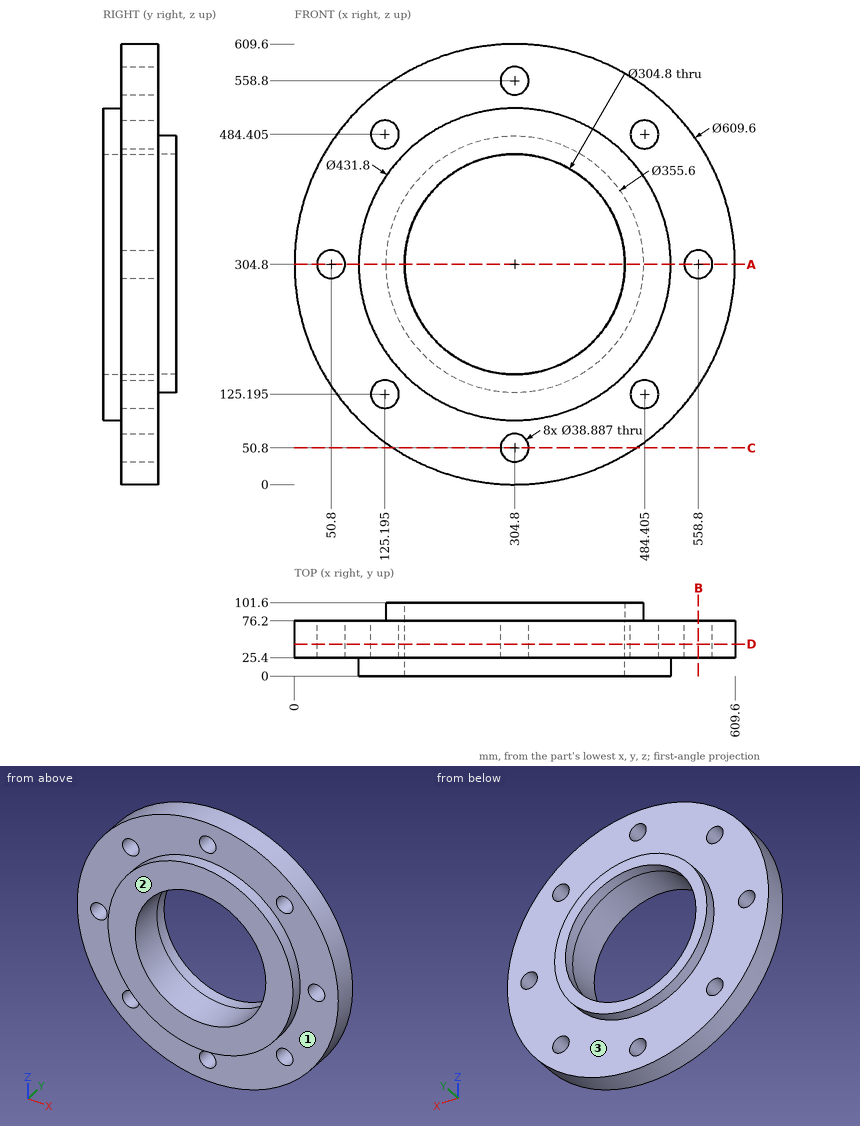
Could you check a few things on this drawing? It's one solid part, dimensions in mm from its lowest x, y, z. A direction names the side the tool comes from. Coordinates: 2 decimals unless noted, no trailing zeros. Order: outer loops, then holes, each group sorted by start corner. A loop starts at its lowest first (then second) coordinate and runs counter-clockwise, first axis right, second up.
1. If we section it at C-C (z = 50.8): Please give me the cut outline in (x, y) (1 decimal), then the cut area to 3 significant figures.
2. If we section it at D-D (y = 44): Give the number of separate pieces and of enclosed holes in the cut face, then the cut area to 3 significant figures.
3. If we section it at A-A (z = 304.8): Please give me the cut outline in (x, y).
4. I'm going to push flat-ended pins straight in: pin 1 (4 mm diameter, centred on x = 467.5, y = 31, fed in from +Z) (1 decimal); pin 2 (5 mm diameter, centred on y = 76, z = 439.5, fed in from -X); pin 3 (5 mm diameter, centred on y = 66.5, z = 245, fed in from -X) (1 decimal); pin 4 (23.5 mm diameter, centred on x = 484.41, z = 125.19, fed in from +Y). Where does each tip first touch, or does it pass through?
5. If we section it at B-B (x = 558.8): Please give me the cut outline in (y, z) (1 decimal).
6. I need wall thicknesses on line 1 (Z direction, x = 373, y = 51); line 2 (Z direction, x = 272, y = 34); line 3 (X direction, y = 42, z = 43.5) (1 decimal). Which ranges of each line are inside material? Lowest first, please.
7. For the marked faces 1, 2 and 3, which set-ups out of +Z, -Z, +X, -X, +Y, -Y let a thin tool reach every point of the face, with its end or its side?
Entries:
1. outline: (136.3, 25.4) - (285.4, 25.4) - (285.4, 76.2) - (136.3, 76.2) - close; (324.2, 25.4) - (473.3, 25.4) - (473.3, 76.2) - (324.2, 76.2) - close
1. area: 15,100 mm2
2. separate pieces: 1
2. enclosed holes: 9
2. area: 209,000 mm2
3. outline: (0, 25.4) - (31.36, 25.4) - (31.36, 76.2) - (0, 76.2) - close; (70.24, 25.4) - (88.9, 25.4) - (88.9, 0) - (152.4, 0) - (152.4, 101.6) - (127, 101.6) - (127, 76.2) - (70.24, 76.2) - close; (457.2, 0) - (520.7, 0) - (520.7, 25.4) - (539.36, 25.4) - (539.36, 76.2) - (482.6, 76.2) - (482.6, 101.6) - (457.2, 101.6) - close; (578.24, 25.4) - (609.6, 25.4) - (609.6, 76.2) - (578.24, 76.2) - close
4. pin 1: stops at z = 563.8
4. pin 2: stops at x = 30.16
4. pin 3: stops at x = 5.4
4. pin 4: passes through
5. outline: (25.4, 136.3) - (76.2, 136.3) - (76.2, 285.4) - (25.4, 285.4) - close; (25.4, 324.2) - (76.2, 324.2) - (76.2, 473.3) - (25.4, 473.3) - close
6. line 1: z = 7.73 to 168.51, 441.09 to 601.87
6. line 2: z = 1.77 to 155.97, 453.63 to 607.83
6. line 3: x = 147.9 to 286.8, 322.8 to 461.7
7. face 1: -Y
7. face 2: +Z, -Z, +X, -X, -Y
7. face 3: +Y
